Check sheet for the modelled part. Datum: model origin and axes. Units: mm. Face numbers are marked on the shaded views. Round coordinates to 2 decimals unless told otherwise and drop trailing zeros. Order: outer loops, then holes, each group sorted by start corner. A loop starts at its lowest first (then second) coordinate and runs counter-clockwise, first axis right, second up.
```python
from build123d import *

# Parameters (mm, degrees)
F0_W     = 152.4
F0_H     = 85.09
F1_DEPTH = 2.54
F2_W     = 152.4
F2_H     = 85.09
F2_W_2   = 149.86
F2_H_2   = 82.55
F3_DEPTH = 1.016
F4_R     = 1.524
F5_DEPTH = 25.4


with BuildPart() as f1:
    # F0 (on Top) → F1 (new body)
    with BuildSketch(Plane.XY):
        Rectangle(F0_W, F0_H)
    extrude(amount=F1_DEPTH)

    # F2 (on face) → F3 (join)
    with BuildSketch(Plane.XY.offset(2.54)):
        Rectangle(F2_W, F2_H)
        Rectangle(F2_W_2, F2_H_2, mode=Mode.SUBTRACT)
    extrude(amount=F3_DEPTH)

    # F4 (on face) → F5 (cut)
    with BuildSketch(Plane.XY.offset(2.54)):
        with Locations((69.215, 35.56)):
            Circle(F4_R)
        with Locations((69.215, -35.56)):
            Circle(F4_R)
        with Locations((-69.215, 35.56)):
            Circle(F4_R)
        with Locations((-69.215, -35.56)):
            Circle(F4_R)
    extrude(amount=-F5_DEPTH, mode=Mode.SUBTRACT)


solid = f1.part
```
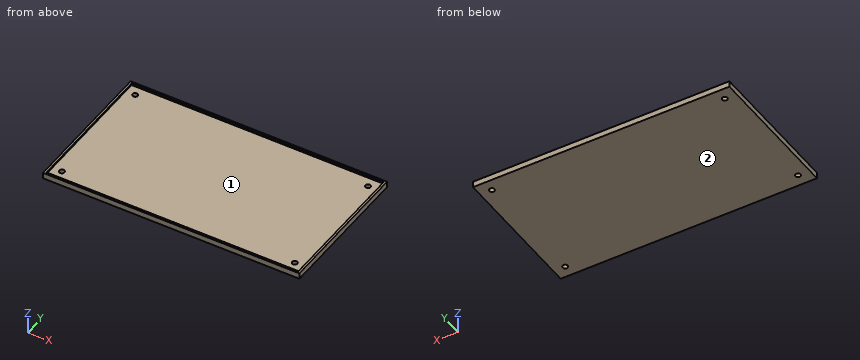
Item 1: Sectioned sample at B-B (x = 46). Record the cut outline in (y, z) (3 decimals), and give its area (3 significant figures).
Answer:
outline: (-42.545, 0) - (42.545, 0) - (42.545, 3.556) - (41.275, 3.556) - (41.275, 2.54) - (-41.275, 2.54) - (-41.275, 3.556) - (-42.545, 3.556) - close
area: 219 mm2
Item 2: Go/stop test with a flat-tipped pin: P1, Ø8, axis at x = 31, y = 5, coming from the +Z side. Record where the tip stops, or that it passes through.
Answer:
P1: stops at z = 2.54
Item 3: Sectioned sample at C-C (y = 5). Record the cut outline in (x, z).
Answer:
outline: (-76.2, 0) - (76.2, 0) - (76.2, 3.56) - (74.93, 3.56) - (74.93, 2.54) - (-74.93, 2.54) - (-74.93, 3.56) - (-76.2, 3.56) - close
Item 4: Sectioned sample at A-A (y = 35.56). Record the cut outline in (x, z).
Answer:
outline: (-76.2, 0) - (-70.74, 0) - (-70.74, 2.54) - (-74.93, 2.54) - (-74.93, 3.56) - (-76.2, 3.56) - close; (-67.69, 0) - (67.69, 0) - (67.69, 2.54) - (-67.69, 2.54) - close; (70.74, 0) - (76.2, 0) - (76.2, 3.56) - (74.93, 3.56) - (74.93, 2.54) - (70.74, 2.54) - close
Item 5: Scan lines: line 1 along Y through (x, z) = (-69, 2.4) (3 decimals); line 2 along Y through (x, z) = (-31, 3.1) (3 decimals); line 3 along X through (y, z) = (-25, 3.05). Record each from-to range of solid material in increasing order.
Answer:
line 1: y = -42.545 to -37.069, -34.051 to 34.051, 37.069 to 42.545
line 2: y = -42.545 to -41.275, 41.275 to 42.545
line 3: x = -76.2 to -74.93, 74.93 to 76.2
Item 6: Release check for a two-part mould opening along X. For the marked faces 1 and 2 record: released by +X, released by -X, zero draft, split by the parting line, or undercut.
Answer:
face 1: undercut
face 2: zero draft
